Could you check a few things on this model? Use its own coordinates, in mm. A direction names the side the tool comes from. Round coordinates to 2 decimals unless told otherwise and drop trailing zeros. Order: outer loops, then holes, each group sorted by start corner. A loop starts at its lowest first (then second) coordinate and runs counter-clockwise, first axis right, second up. Notation, with made-up numbers: M 66.25,35.25 L 116.25,35.25 A14 cw 116.25,40.25 Z; hole C 4,48.25 d2. An arc over 180 degrees is marked long. Write each question's results on one line, items separated by ' | '. Start each with the question number.
1. I'm going to push flat-ended pins straight in: pin 1 (17.5 mm diameter, centred on x = -11, y = 110, fed in from +Z); pin 2 (6.5 mm diameter, centred on x = -13, z = 10.5, fed in from +Y). Where does each tip first touch, or does it pass through?
2. We'd pull the mould along X, two halves only. Please class faces 3 (the flat face through (32.5, 102, 9)), 4 (the flat face through (115, 2, 6)), 5 (the flat face through (-2, -23, 12)): released by +X, released by -X, zero draft, split by the parting line, or undercut.
3. Please list where these lines run through material, in increasing order: L1, parallel to Y at x = 25, z = 10; L2, parallel to Y at x = -77.5, z = 4.25 (3 decimals); L3, parallel to X at y = -134, z = 8.5.
4. Suppose I cut it at B-B on x = -19.5. Write out the boundary of the cut face in (y, z).
5. For faces 1 (the flat face through (-115, -2, 6)), 2 (the flat face through (-32.5, 102, 9)), which set-ups out of +Z, -Z, +X, -X, +Y, -Y let a thin tool reach every point of the face, with its end or its side?
6. Suppose I cut it at C-C on y = -128. Write out the boundary of the cut face in (x, z).
7. Suppose I cut it at A-A on z = 9.5. Write out the boundary of the cut face in (x, y).
8. Suppose I cut it at D-D on x = 85.5. Write out the boundary of the cut face in (y, z) (3 decimals), and give its area (3 significant figures).
from build123d import *

# Parameters (mm, degrees)
BOSS_EXTRUDE1_DEPTH   = 13.1
FILLET1_R             = 5
SKETCH2_W             = 65
SKETCH2_H             = 35
CUT_EXTRUDE1_DEPTH    = 206.661396475
SKETCH3_W             = 109.473839025
SKETCH3_H             = 48.944636842
BOSS_EXTRUDE2_DEPTH   = 7
BODY_MOVE_COPY1_ANGLE = 180
DELETEFACE1_START     = -1.1
DELETEFACE1_DEPTH     = 13.1


# Read off the part's stored shape, not the designer's step: DeleteFace1
with BuildPart() as part:
    # Sketch1 → Boss-Extrude1 (new body)
    with BuildSketch(Plane.XY):
        Polygon((115, -120), (115, 120), (-115, 120), (-115, -120), (-75, -170), (75, -170), align=None)
    extrude(amount=BOSS_EXTRUDE1_DEPTH)

    # Fillet1
    fillet1_edges = [part.edges().sort_by_distance(p)[0] for p in [
        (-115, 120, 6.55),
        (115, 120, 6.55),
        (115, -120, 6.55),
        (75, -170, 6.55),
        (-75, -170, 6.55),
        (-115, -120, 6.55),
    ]]
    fillet(fillet1_edges, radius=FILLET1_R)

    # Sketch2 → Cut-Extrude1 (cut, through all)
    with BuildSketch(Plane.XY.offset(13.1)):
        with Locations((0, 102.5)):
            Rectangle(SKETCH2_W, SKETCH2_H)
    extrude(amount=-CUT_EXTRUDE1_DEPTH, mode=Mode.SUBTRACT)

    # Sketch3 → Boss-Extrude2 (add)
    with BuildSketch(Plane.XY.offset(13.1)):
        with Locations((2.558327619, 95.527681579)):
            Rectangle(SKETCH3_W, SKETCH3_H)
    extrude(amount=-BOSS_EXTRUDE2_DEPTH)


with BuildPart() as part_1:
    # Body-Move/Copy1: moved
    add(part.part.rotate(Axis((0, 0, 6), (0, 1, 0)), BODY_MOVE_COPY1_ANGLE))

    # DeleteFace1 outline → DeleteFace1 (add)
    with BuildSketch(Plane.XY.offset(DELETEFACE1_START)):
        with BuildLine():
            ThreePointArc((-72.596875763, -170), (-74.762819415, -169.506516182), (-76.50121981, -168.123475238))
            Line((-76.50121981, -168.123475238), (-75, -170))
            Line((-75, -170), (-72.596875763, -170))
        make_face()
        with BuildLine():
            Line((-115, -120), (-113.904344047, -121.369569941))
            ThreePointArc((-113.904344047, -121.369569941), (-114.718141596, -119.90112941), (-115, -118.246094703))
            Line((-115, -118.246094703), (-115, -120))
        make_face()
        with BuildLine():
            ThreePointArc((76.50121981, -168.123475238), (74.762819415, -169.506516182), (72.596875763, -170))
            Line((72.596875763, -170), (75, -170))
            Line((75, -170), (76.50121981, -168.123475238))
        make_face()
        with BuildLine():
            Line((-115, 120), (-115, 115))
            ThreePointArc((-115, 115), (-113.535533906, 118.535533906), (-110, 120))
            Line((-110, 120), (-115, 120))
        make_face()
        with BuildLine():
            ThreePointArc((115, -118.246094703), (114.718141596, -119.90112941), (113.904344047, -121.369569941))
            Line((113.904344047, -121.369569941), (115, -120))
            Line((115, -120), (115, -118.246094703))
        make_face()
        with BuildLine():
            Line((115, 120), (110, 120))
            ThreePointArc((110, 120), (113.535533906, 118.535533906), (115, 115))
            Line((115, 115), (115, 120))
        make_face()
    extrude(amount=DELETEFACE1_DEPTH)


solid = part_1.part
Filled sheet:
1) pin 1: stops at z = 5.9 | pin 2: stops at y = 85
2) face 3: undercut | face 4: released by +X | face 5: zero draft
3) L1: y = -170 to 85 | L2: y = -166.875 to 120 | L3: x = -103.8 to 103.8
4) outline: M -170,-1.1 L 120,-1.1 L 120,5.9 L 85,5.9 L 85,12 L -170,12 Z
5) face 1: +Z, -Z, -X, +Y, -Y | face 2: +Z, +Y
6) outline: M -108.6,-1.1 L 108.6,-1.1 L 108.6,12 L -108.6,12 Z
7) outline: M -115,-120 L -75,-170 L 75,-170 L 115,-120 L 115,120 L 32.5,120 L 32.5,85 L -32.5,85 L -32.5,120 L -115,120 Z
8) outline: M -156.875,-1.1 L 120,-1.1 L 120,12 L -156.875,12 Z | area: 3,630 mm^2
